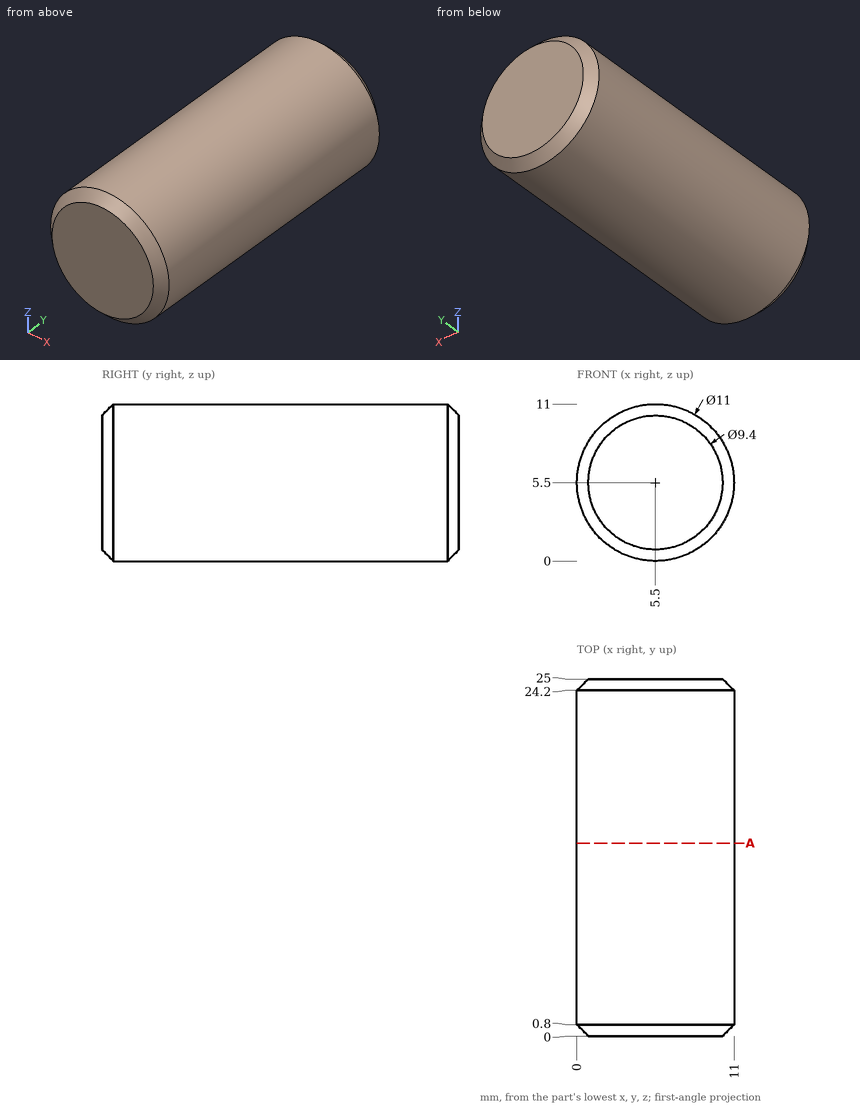
Check sheet for the drawn part. Datum: minimum x, y, z corner. Units: mm. Round coordinates to 2 decimals unless told otherwise and drop trailing zeros. Loops run counter-clockwise (first coordinate to the right, second up) from the corner with the lowest first, then second, coordinate; pieces in that order, holes last. Notation, with made-up numbers: M -29.5,78 L -0.5,78 A23 ccw -0.5,115 Z; hole C -8,21.5 d8. An arc over 180 degrees is marked long. One line per question, with ' | ' between items. Start each with the question number.
Item 1: Section check A-A (y = 13.5). Record the boundary of the cut face in (x, z), and give its area (3 significant figures).
Item 2: Gauge pin test, flat ends, axial feed: pin 1 Ø1 at (x, z) = (9.5, 2) entering from -Y; pin 2 Ø1.5 at (y, z) = (13.5, 2) entering from +X; pin 3 Ø4 at (y, z) = (4.5, 3) entering from -X; pin 4 Ø2 at (x, z) = (3.5, 4.5) entering from -Y. Record the tip position at first contact, or that the pin passes through.
Item 3: Scan lines: probe 1 along X at (y, z) = (20.25, 1.5); probe 2 along Z at (x, y) = (9.75, 11); probe 3 along X at (y, z) = (18.75, 8.75). Record each from-to range of solid material in increasing order.
Worked out:
1) outline: C 5.5,5.5 d11 | area: 95.0 mm^2
2) pin 1: y = 0.12 | pin 2: x = 10.26 | pin 3: x = 0.02 | pin 4: y = 0
3) probe 1: 1.73 to 9.27 | probe 2: 2.01 to 8.99 | probe 3: 1.06 to 9.94
